Check sheet for the modelled part. Datum: model origin and axes. Units: mm. A direction names the side the tool comes from. Coordinates: 2 decimals unless noted, no trailing zeros. Write each loop counter-clockwise with the first axis right and the second up, starting at its lowest first coordinate (ties: lowest second). Pieces come first, ordered by that corner, then holes. Notation, with made-up numbers: M -36.75,83 L 1.25,83 A30 cw 1.25,107 Z; hole C 26,53 d7. An arc over 180 degrees is marked long. Answer as CSV lines item,"result".
from build123d import *

# Parameters (mm, degrees)
BOSS_EXTRUDE1_DEPTH = 36
SKETCH2_R           = 3
CUT_EXTRUDE1_DEPTH  = 5
SKETCH3_R           = 3
CUT_EXTRUDE2_DEPTH  = 5
FILLET1_R           = 5


with BuildPart() as part:
    # Sketch1 → Boss-Extrude1 (new body)
    with BuildSketch(Plane.XY):
        Polygon((0, 19.095465902), (0, -0.904534098), (30, -0.904534098), (30, -5.904534098), (-5, -5.904534098), (-5, 19.095465902), align=None)
    extrude(amount=BOSS_EXTRUDE1_DEPTH)

    # Sketch2 → Cut-Extrude1 (cut)
    with BuildSketch(Plane(origin=(0, -0.904534098, 0), x_dir=(1, 0, 0), z_dir=(0, 1, 0))):
        with Locations(Location((22, -8, 0), (0, 0, 180))):
            Circle(SKETCH2_R)
        with Locations(Location((22, -28, 0), (0, 0, 180))):
            Circle(SKETCH2_R)
    extrude(amount=-CUT_EXTRUDE1_DEPTH, mode=Mode.SUBTRACT)

    # Sketch3 → Cut-Extrude2 (cut)
    with BuildSketch(Plane(origin=(0, 0, 0), x_dir=(0, 0, -1), z_dir=(1, 0, 0))):
        with Locations(Location((-28, 7.095465902, 0), (0, 0, 90))):
            Circle(SKETCH3_R)
        with Locations(Location((-8, 7.095465902, 0), (0, 0, 90))):
            Circle(SKETCH3_R)
    extrude(amount=-CUT_EXTRUDE2_DEPTH, mode=Mode.SUBTRACT)

    # Fillet1
    fillet1_edges = [part.edges().sort_by_distance(p)[0] for p in [
        (30, -3.404534098, 36),
        (-2.5, 19.095465902, 36),
        (30, -3.404534098, 0),
        (-2.5, 19.095465902, 0),
    ]]
    fillet(fillet1_edges, radius=FILLET1_R)


solid = part.part
1) Depth check by flat-ended pin: P1, Ø1.5, axis at x = 12, z = 27, coming from the +Y side; P2, Ø3.5, axis at y = 7.1, z = 28, coming from the -X side. Enter the tip coordinate at first touch or a pass-through.
Answer key:
P1,"stops at y = -0.9"
P2,"passes through"
2) Thickness scan on line 1 along Z through (x, y) = (22, -2.8); line 2 along Y through (x, z) = (2.5, 30); line 3 along X through (y, z) = (16.75, 12). Record the ranges inside material, lowest first.
Answer key:
line 1,"z = 0 to 5, 11 to 25, 31 to 36"
line 2,"y = -5.9 to -0.9"
line 3,"x = -5 to 0"
3) Section check A-A, the plane x = 22. Record the boundary of the cut face in (y, z), plus the area to 3 significant figures.
Answer key:
outline,"M -5.9,0 L -0.9,0 L -0.9,5 L -5.9,5 Z; M -5.9,11 L -0.9,11 L -0.9,25 L -5.9,25 Z; M -5.9,31 L -0.9,31 L -0.9,36 L -5.9,36 Z"
area,"120 mm2"
4) Section check D-D, the plane y = 13. Record the boundary of the cut face in (x, z), plus the area to 3 significant figures.
Answer key:
outline,"M -5,0 L 0,0 L 0,36 L -5,36 Z"
area,"180 mm2"
5) Section check C-C, the plane z = 16.5. Record the boundary of the cut face in (x, y).
Answer key:
outline,"M -5,-5.9 L 30,-5.9 L 30,-0.9 L 0,-0.9 L 0,19.1 L -5,19.1 Z"
6) Section check B-B, the plane z = 8. Record the boundary of the cut face in (x, y), plus the area to 3 significant figures.
Answer key:
outline,"M -5,-5.9 L 19,-5.9 L 19,-0.9 L 0,-0.9 L 0,4.1 L -5,4.1 Z; M -5,10.1 L 0,10.1 L 0,19.1 L -5,19.1 Z; M 25,-5.9 L 30,-5.9 L 30,-0.9 L 25,-0.9 Z"
area,"215 mm2"
7) Mould release check, pull along X, two halves, no side actions. Record for faces 3 (the face through (30, -3, 18)), 4 (the face through (-2.465, 9.957, 28.901)), 5 (the face through (25, -3, 8)), 6 (the face through (25, -3, 28)): pulls with the +X half, pulls with the -X half, needs draft (parallel to the pull), parting line crosses it, or undercut.
Answer key:
face 3,"pulls with the +X half"
face 4,"needs draft"
face 5,"undercut"
face 6,"undercut"
8) Tool access check on faces 1 (the face through (13, -5.905, 18)), 2 (the face through (15, -0.905, 18)). Record the directions out of +Z, -Z, +X, -X, +Y, -Y that give a thin tool (end or side, any length) a straight path to the whole face; none if there is none.
Answer key:
face 1,"+Z, -Z, +X, -X, -Y"
face 2,"+Z, -Z, +X, +Y"
